Check sheet for the modelled part. Datum: model origin and axes. Units: mm. A direction names the side the tool comes from. Give positions to 0.01 mm unless a question says otherwise; leave off trailing zeros. Order: outer loops, then holes, each group sorted by start corner. A loop starts at its lowest first (then second) coordinate and runs counter-clockwise, first axis right, second up.
```python
from build123d import *

# Parameters (mm, degrees)
SKETCH1_W                                   = 53.2
SKETCH1_H                                   = 21.5
BOSS_EXTRUDE1_DEPTH                         = 12
SKETCH2_R                                   = 0.9
CUT_EXTRUDE1_DEPTH                          = 5
SKETCH3_W                                   = 6
SKETCH3_H                                   = 8.5
CUT_EXTRUDE2_DEPTH                          = 13
SKETCH5_R                                   = 2
CUT_EXTRUDE3_DEPTH                          = 1.5
CBORE_FOR_M3_CHEESE_HEAD_SCREW1_D           = 3.4
CBORE_FOR_M3_CHEESE_HEAD_SCREW1_CBORE_D     = 6.5
CBORE_FOR_M3_CHEESE_HEAD_SCREW1_CBORE_DEPTH = 4
CUT_EXTRUDE4_DEPTH                          = 22.5
FILLET1_R                                   = 5
CHAMFER2_SIZE                               = 0.5
CHAMFER3_SIZE                               = 0.5


with BuildPart() as part:
    # Sketch1 → Boss-Extrude1 (new body)
    with BuildSketch(Plane(origin=(0, 0, 0), x_dir=(1, 0, 0), z_dir=(0, 1, 0))):
        Rectangle(SKETCH1_W, SKETCH1_H)
    extrude(amount=BOSS_EXTRUDE1_DEPTH)

    # Sketch2 → Cut-Extrude1 (cut)
    with BuildSketch(Plane(origin=(0, 12, 0), x_dir=(1, 0, 0), z_dir=(0, 1, 0))):
        with Locations((24.4, 8.25)):
            Circle(SKETCH2_R)
        with Locations((24.4, -8.25)):
            Circle(SKETCH2_R)
        with Locations((-10.6, -8.25)):
            Circle(SKETCH2_R)
        with Locations((-10.6, 8.25)):
            Circle(SKETCH2_R)
    extrude(amount=-CUT_EXTRUDE1_DEPTH, mode=Mode.SUBTRACT)

    # Sketch3 → Cut-Extrude2 (cut, through all)
    with BuildSketch(Plane.XZ):
        with Locations((23.6, 0)):
            Rectangle(SKETCH3_W, SKETCH3_H)
    extrude(amount=-CUT_EXTRUDE2_DEPTH, mode=Mode.SUBTRACT)

    # Sketch5 → Cut-Extrude3 (cut)
    with BuildSketch(Plane(origin=(0, 12, 0), x_dir=(1, 0, 0), z_dir=(0, 1, 0))):
        with Locations((-19.85, 7.25)):
            Circle(SKETCH5_R)
        with Locations((-19.85, -7.25)):
            Circle(SKETCH5_R)
        with BuildLine():
            Line((-0.75, -3.85), (4.85, -3.85))
            ThreePointArc((4.85, -3.85), (6.35, -5.35), (4.85, -6.85))
            Line((4.85, -6.85), (-0.75, -6.85))
            ThreePointArc((-0.75, -6.85), (-2.25, -5.35), (-0.75, -3.85))
        make_face()
    extrude(amount=-CUT_EXTRUDE3_DEPTH, mode=Mode.SUBTRACT)

    # CBORE for M3 Cheese Head Screw1 (through all)
    with Locations(Plane(origin=(-11.6, 12, 0), x_dir=(0, 0, 1), z_dir=(0, 1, 0))):
        with Locations((0, 0), (0, 23)):
            CounterBoreHole(CBORE_FOR_M3_CHEESE_HEAD_SCREW1_D / 2, CBORE_FOR_M3_CHEESE_HEAD_SCREW1_CBORE_D / 2, CBORE_FOR_M3_CHEESE_HEAD_SCREW1_CBORE_DEPTH)

    # Sketch9 → Cut-Extrude4 (cut, through all)
    with BuildSketch(Plane.XY.offset(10.75)):
        Polygon((-17.486751346, 10), (-26.6, 10), (-26.6, 0), (-14.6, 0), (-14.6, 5), align=None)
        Polygon((5.513248654, 10), (-5.713248654, 10), (-8.6, 5), (-8.6, 0), (8.4, 0), (8.4, 5), align=None)
        Polygon((26.6, 0), (26.6, 10), (17.286751346, 10), (14.4, 5), (14.4, 0), align=None)
    extrude(amount=-CUT_EXTRUDE4_DEPTH, mode=Mode.SUBTRACT)

    # Fillet1
    fillet1_edges = [part.edges().sort_by_distance(p)[0] for p in [
        (-14.6, 5, 0),
        (-17.486751346, 10, 0),
        (8.4, 5, 0),
        (-8.6, 5, 0),
        (-5.713248654, 10, 0),
        (5.513248654, 10, 0),
        (17.286751346, 10, 0),
        (14.4, 5, 0),
    ]]
    fillet(fillet1_edges, radius=FILLET1_R)

    # Chamfer2
    chamfer2_edges = [part.edges().sort_by_distance(p)[0] for p in [
        (-11.5, 7, -8.25),
        (-11.5, 7, 8.25),
        (-2.25, 10.5, 5.35),
        (2.05, 10.5, 3.85),
        (6.35, 10.5, 5.35),
        (2.05, 10.5, 6.85),
        (-21.85, 10.5, 7.25),
        (-21.85, 10.5, -7.25),
        (11.4, 8, 1.7),
        (-11.6, 8, 1.7),
    ]]
    chamfer(chamfer2_edges, length=CHAMFER2_SIZE)

    # Chamfer3
    chamfer3_edges = [part.edges().sort_by_distance(p)[0] for p in [
        (-26.6, 12, 0),
        (23.6, 10, -4.25),
        (0, 12, 10.75),
        (26.6, 12, -7.5),
        (20.6, 12, 0),
        (23.6, 12, 4.25),
        (26.6, 12, 7.5),
        (0, 12, -10.75),
    ]]
    chamfer(chamfer3_edges, length=CHAMFER3_SIZE)


solid = part.part
```
(1) Sectioned sample at A-A (y = 1.75). Enter the section's corners in (x, z).
(2) Tool access check on faces 1 (the face through (8.225, 4.972, -0.151)), 2 (the face through (23, 10, 5)), 3 (the face through (26.6, 11, 8)), 4 (the face through (25.26, 11.01, -8.52)), 5 (the face through (2.1, 11.5, 6.85)). Record the directions out of +Z, -Z, +X, -X, +Y, -Y that give a thin tool (end or side, any length) a straight path to the whole face; none if there is none.
(3) Release check for a two-part mould opening along X. For faces 6 (the face through (-2.25, 11.51, 5.38)), 7 (the face through (14.4, 2, 0)), 8 (the face through (-23, 10, 0)) record: released by +X, released by -X, zero draft, split by the parting line, or undercut.
(4) Go/stop test with flat-tipped pins: P1, Ø4, axis at x = 11.4, z = 0, coming from the +Y side; P2, Ø0.8, axis at y = 11, z = -1, coming from the +X side; P3, Ø1.4, axis at x = 24.4, z = 8.25, coming from the -Y side (1 decimal); P4, Ø4, axis at y = 2.5, z = -2.5, coming from the -X side. Record where each tip stops, or that it passes through.
(5) Thickness scan on L1, parallel to X at y = 11.1, z = 0; L2, parallel to Z at x = -19.85, y = 11.65; L3, parallel to X at y = 2.5, z = 7.25. Record the ranges inside material, lowest first.
(6) Sectioned sample at C-C (x = -19.85). Enter the section's corners in (y, z), plus the area to 3 significant figures.
(7) Sectioned sample at B-B (z = 0). Count the separate pieces of the cut face and the enclosed holes in it, plus the area to 3 significant figures.
Values follow:
1. outline: (-14.6, -10.75) - (-8.6, -10.75) - (-8.6, 10.75) - (-14.6, 10.75) - close; (8.4, -10.75) - (14.4, -10.75) - (14.4, 10.75) - (8.4, 10.75) - close; hole circle Ø3.4 at (-11.6, 0); hole circle Ø3.4 at (11.4, 0)
2. face 1: +Z, -Z, -Y
2. face 2: +Z, -Z, +X, -Y
2. face 3: +Z, -Z, +X, +Y, -Y
2. face 4: +Y, -Y
2. face 5: +Y
3. face 6: undercut
3. face 7: released by +X
3. face 8: zero draft
4. P1: stops at y = 7.8
4. P2: stops at x = 20.6
4. P3: passes through
4. P4: stops at x = -14.67
5. L1: x = -26.6 to -14.85, -8.35 to 8.15, 14.65 to 20.6
5. L2: z = -10.6 to -9.25, -5.25 to 5.25, 9.25 to 10.6
5. L3: x = -14.6 to -8.6, 8.4 to 14.4
6. outline: (9.97, -10.75) - (11.5, -10.75) - (12, -10.25) - (12, -9.25) - (11, -9.25) - (10.5, -8.75) - (10.5, -5.75) - (11, -5.25) - (12, -5.25) - (12, 5.25) - (11, 5.25) - (10.5, 5.75) - (10.5, 8.75) - (11, 9.25) - (12, 9.25) - (12, 10.25) - (11.5, 10.75) - (9.97, 10.75) - close
6. area: 31.8 mm2
7. separate pieces: 3
7. enclosed holes: 0
7. area: 142 mm2
